Could you check a few things on this model? Use its own coordinates, in mm. A direction names the side the tool comes from. Round coordinates to 2 decimals unless told otherwise and drop trailing zeros. Write each loop counter-clockwise with the first axis right and the second up, starting at its lowest first coordinate (ties: lowest second). Pieces come first, ordered by that corner, then holes. Notation, with made-up numbers: M -34.5,53 L -16.5,53 A22 cw -16.5,92 Z; hole C 10,-19.5 d10. An arc over 180 degrees is marked long. One line per item, written item: value. Start each with the question number.
(1) Thinking about a two-plate mould opening in X: for faces 4 (the face through (5.57, 23.15, -7)), 5 (the face through (0, 17, -21)), 6 (the face through (21, 0, -19)), which applies, released by +X, released by -X, zero draft, split by the parting line, or undercut?
(2) I want a section at D-D on x = 21. Please give me the cut outline in (y, z), and give its area (3 significant figures).
(3) I want a section at C-C on y = 42. Please give me the cut outline in (x, z).
(4) I'm going to push flat-ended pins straight in: pin 1 Ø3.5 at (x, z) = (5.5, -6) entering from +Y; pin 2 Ø1.8 at (x, z) = (36.5, -5.5) entering from +Y; pin 3 Ø4 at (y, z) = (4.5, 2.5) entering from -X. Where does each tip first touch, or does it pass through?
(5) I want a section at A-A on x = 5.5. Please give me the cut outline in (y, z).
(6) Which directions (+Z, -Z, +X, -X, +Y, -Y) give clear straight access to the entire face, cutting with the end or side of a thin tool? Please do faces 1 (the face through (4.6, 23.2, -37.7)), 2 (the face through (39, 17, -38)), 3 (the face through (29, 5, 2)).
(7) If I drill on L1, parallel to X at y = 35, z = -21; L2, parallel to X at y = 26.75, z = -36.5; L3, parallel to Z at x = 5, y = 23, over which ranges is the centre line in solid material (lowest first)?
(8) I want a section at B-B on z = -21. Please give me the cut outline in (x, y).
```python
from build123d import *

# Parameters (mm, degrees)
BOSS_EXTRUDE1_DEPTH = 34
SKETCH2_W           = 16
SKETCH2_H           = 10
BOSS_EXTRUDE2_DEPTH = 5
SKETCH3_R           = 11
SKETCH3_R_2         = 5
BOSS_EXTRUDE3_DEPTH = 2
SKETCH4_R           = 2.5
BOSS_EXTRUDE4_DEPTH = 22
SKETCH5_R           = 1.5
CUT_EXTRUDE1_DEPTH  = 22


with BuildPart() as part:
    # Sketch1 → Boss-Extrude1 (new body)
    with BuildSketch(Plane(origin=(0, 0, 0), x_dir=(1, 0, 0), z_dir=(0, 1, 0))):
        Polygon((7, 42), (0, 35), (0, 7), (7, 0), (35, 0), (42, 7), (42, 35), (35, 42), align=None)
    extrude(amount=BOSS_EXTRUDE1_DEPTH)

    # Sketch2 → Boss-Extrude2 (add)
    with BuildSketch(Plane.XY):
        with Locations((21, 5)):
            Rectangle(SKETCH2_W, SKETCH2_H)
    extrude(amount=BOSS_EXTRUDE2_DEPTH)

    # Sketch3 → Boss-Extrude3 (add)
    with BuildSketch(Plane(origin=(0, 34, 0), x_dir=(1, 0, 0), z_dir=(0, 1, 0))):
        with Locations(Location((21, 21, 0), (0, 0, 270))):
            Circle(SKETCH3_R)
        with Locations(Location((21, 21, 0), (0, 0, 270))):
            Circle(SKETCH3_R_2, mode=Mode.SUBTRACT)
    extrude(amount=BOSS_EXTRUDE3_DEPTH)

    # Sketch4 → Boss-Extrude4 (add)
    with BuildSketch(Plane(origin=(0, 34, 0), x_dir=(1, 0, 0), z_dir=(0, 1, 0))):
        with Locations(Location((21, 21, 0), (0, 0, 270))):
            Circle(SKETCH4_R)
    extrude(amount=BOSS_EXTRUDE4_DEPTH)

    # Sketch5 → Cut-Extrude1 (cut)
    with BuildSketch(Plane(origin=(0, 34, 0), x_dir=(1, 0, 0), z_dir=(0, 1, 0))):
        with Locations(Location((5.5, 36.5, 0), (0, 0, 270))):
            Circle(SKETCH5_R)
        with Locations(Location((5.5, 5.5, 0), (0, 0, 270))):
            Circle(SKETCH5_R)
        with Locations(Location((36.5, 5.5, 0), (0, 0, 270))):
            Circle(SKETCH5_R)
        with Locations(Location((36.5, 36.5, 0), (0, 0, 270))):
            Circle(SKETCH5_R)
    extrude(amount=-CUT_EXTRUDE1_DEPTH, mode=Mode.SUBTRACT)


solid = part.part
```
Found:
1. face 4: undercut
1. face 5: released by -X
1. face 6: zero draft
2. outline: M 0,-42 L 34,-42 L 34,-32 L 36,-32 L 36,-26 L 34,-26 L 34,-23.5 L 56,-23.5 L 56,-18.5 L 34,-18.5 L 34,-16 L 36,-16 L 36,-10 L 34,-10 L 34,0 L 10,0 L 10,5 L 0,5 Z
2. area: 1,610 mm²
3. outline: C 21,-21 d5
4. pin 1: stops at y = 34
4. pin 2: stops at y = 12
4. pin 3: stops at x = 13
5. outline: M 0,-40.5 L 34,-40.5 L 34,-38 L 12,-38 L 12,-35 L 34,-35 L 34,-7 L 12,-7 L 12,-4 L 34,-4 L 34,-1.5 L 0,-1.5 Z
6. face 1: +Y
6. face 2: -Z, +X, +Y, -Y
6. face 3: +Z, +X, +Y, -Y
7. L1: x = 10 to 16, 18.5 to 23.5, 26 to 32
7. L2: x = 1.5 to 4, 7 to 35, 38 to 40.5
7. L3: z = -40 to -37.91, -35.09 to -6.91, -4.09 to -2
8. outline: M 0,0 L 42,0 L 42,34 L 32,34 L 32,36 L 26,36 L 26,34 L 23.5,34 L 23.5,56 L 18.5,56 L 18.5,34 L 16,34 L 16,36 L 10,36 L 10,34 L 0,34 Z
